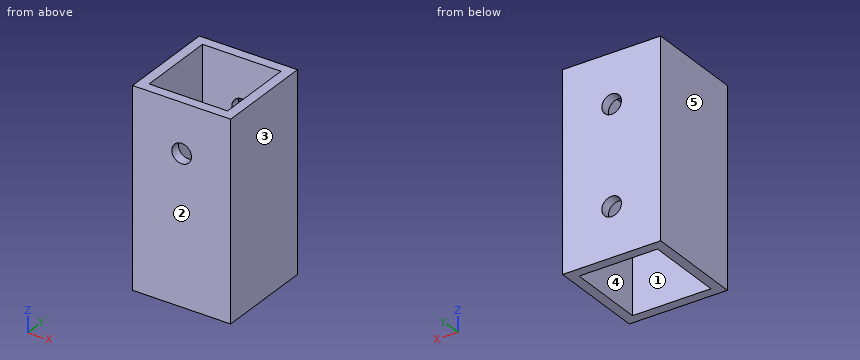
from build123d import *

# Parameters (mm, degrees)
SKETCH_1_W          = 15
SKETCH_1_H          = 15
SKETCH_1_W_2        = 12
SKETCH_1_H_2        = 12
EXTRUDE_2_DEPTH     = 30
SKETCH_2_R          = 1.5
CUT_EXTRUDE_1_DEPTH = 20
SKETCH_3_R          = 1.5
CUT_EXTRUDE_2_DEPTH = 10


with BuildPart() as part:
    # ｽｹｯﾁ1 → ﾎﾞｽ - 押し出し2 (new body)
    with BuildSketch(Plane.XY):
        with Locations((0.489915859, 0.232626086)):
            Rectangle(SKETCH_1_W, SKETCH_1_H)
        with Locations((0.489915859, 0.232626086)):
            Rectangle(SKETCH_1_W_2, SKETCH_1_H_2, mode=Mode.SUBTRACT)
    extrude(amount=EXTRUDE_2_DEPTH)

    # ｽｹｯﾁ2 → ｶｯﾄ - 押し出し1 (cut)
    with BuildSketch(Plane(origin=(0, 7.732626086, 0), x_dir=(1, 0, 0), z_dir=(0, 1, 0))):
        with Locations((0.489915859, -22.5)):
            Circle(SKETCH_2_R)
    extrude(amount=-CUT_EXTRUDE_1_DEPTH, mode=Mode.SUBTRACT)

    # ｽｹｯﾁ3 → ｶｯﾄ - 押し出し2 (cut)
    with BuildSketch(Plane(origin=(0, 7.732626086, 0), x_dir=(1, 0, 0), z_dir=(0, 1, 0))):
        with Locations((0.489915859, -7.5)):
            Circle(SKETCH_3_R)
    extrude(amount=-CUT_EXTRUDE_2_DEPTH, mode=Mode.SUBTRACT)


solid = part.part
Model file for the job. Use its own axes, mm. Face numbers are marked on the shaded views. A direction names the side the tool comes from. Give positions to 0.01 mm unless a question says otherwise; leave off trailing zeros. Order: outer loops, then holes, each group sorted by start corner. A loop starts at its lowest first (then second) coordinate and runs counter-clockwise, first axis right, second up. Notation, with made-up numbers: (49, 64) - (75, 64) arc R12 ccw to (75, 79) - close; hole circle Ø3 at (8, -25.5). An arc over 180 degrees is marked (long way). Return JSON: item names as keys, results as strings.
1) Flat gauge pin, fed straight in: P1, Ø4, axis at x = 0, y = 3, coming from the -Z side. Where does the tip first touch, or does it go through?
Geometry says:
{"P1": "through"}
2) Cut at D-D, the plane z = 7.5. Give the cut face in (x, y).
Geometry says:
{"outline": "(-7.01, -7.27) - (7.99, -7.27) - (7.99, 7.73) - (1.99, 7.73) - (1.99, 6.23) - (6.49, 6.23) - (6.49, -5.77) - (-5.51, -5.77) - (-5.51, 6.23) - (-1.01, 6.23) - (-1.01, 7.73) - (-7.01, 7.73) - close"}
3) Pull direction Y, two halves, no side cores. Call the marked faces 1, 2 and 3: pulls with the +Y half, pulls with the -Y half, needs draft (parallel to the pull), parting line crosses it, or undercut.
Geometry says:
{"face 1": "undercut", "face 2": "pulls with the -Y half", "face 3": "needs draft"}
4) Cut at B-B, the plane y = -1. Give the cut face in (x, z), plus the area to 3 significant figures.
Geometry says:
{"outline": "(-7.01, 0) - (-5.51, 0) - (-5.51, 30) - (-7.01, 30) - close; (6.49, 0) - (7.99, 0) - (7.99, 30) - (6.49, 30) - close", "area": "90.0 mm²"}
5) Cut at C-C, the plane z = 22.5. Give the cut face in (x, y).
Geometry says:
{"outline": "(-7.01, -7.27) - (-1.01, -7.27) - (-1.01, -5.77) - (-5.51, -5.77) - (-5.51, 6.23) - (-1.01, 6.23) - (-1.01, 7.73) - (-7.01, 7.73) - close; (1.99, -7.27) - (7.99, -7.27) - (7.99, 7.73) - (1.99, 7.73) - (1.99, 6.23) - (6.49, 6.23) - (6.49, -5.77) - (1.99, -5.77) - close"}
6) Probe line 1 (X direction, y = -6.55, z = 22.5); line 2 (Y direction, x = -2, z = 13.5); line 3 (X direction, y = 6, z = 5.5). List the from-to ranges inside material, lowest first. Write a range as from..to.
Geometry says:
{"line 1": "-7.01..-1.01, 1.99..7.99", "line 2": "-7.27..-5.77, 6.23..7.73", "line 3": "-7.01..-5.51, 6.49..7.99"}
7) 3-axis set-ups, long thin cutter, end or side, ignore diameter. For the marked faces 4 and 5: which of +Z, -Z, +X, -X, +Y, -Y reach the whole face in a straight line?
Geometry says:
{"face 4": "+Z, -Z", "face 5": "+Z, -Z, -X, +Y, -Y"}
8) Cut at A-A, the plane z = 3.5. Give the cut face in (x, y).
Geometry says:
{"outline": "(-7.01, -7.27) - (7.99, -7.27) - (7.99, 7.73) - (-7.01, 7.73) - close; hole (-5.51, -5.77) - (6.49, -5.77) - (6.49, 6.23) - (-5.51, 6.23) - close"}
